```python
from build123d import *

# Parameters (mm, degrees)
EXTRUDE_1_DEPTH     = 2.5
CUT_EXTRUDE_1_DEPTH = 1
CUT_EXTRUDE_2_DEPTH = 3.8
CUT_EXTRUDE_3_DEPTH = 1


with BuildPart() as part:
    # Sketch 1 → Extrude 1 (new body)
    with BuildSketch(Plane(origin=(0, 0, 0), x_dir=(1, 0, 0), z_dir=(0, 1, 0))):
        Polygon((-33.25966317, -13.776603565), (-13.776603565, -33.25966317), (13.776603565, -33.25966317), (33.25966317, -13.776603565), (33.25966317, 13.776603565), (13.776603565, 33.25966317), (-13.776603565, 33.25966317), (-33.25966317, 13.776603565), align=None)
        Polygon((-13.27954729, -32.05966317), (13.27954729, -32.05966317), (32.05966317, -13.27954729), (32.05966317, 13.27954729), (13.27954729, 32.05966317), (-13.27954729, 32.05966317), (-32.05966317, 13.27954729), (-32.05966317, -13.27954729), align=None, mode=Mode.SUBTRACT)
        Polygon((-32.05966317, -13.27954729), (-13.27954729, -32.05966317), (13.27954729, -32.05966317), (32.05966317, -13.27954729), (32.05966317, 13.27954729), (13.27954729, 32.05966317), (-13.27954729, 32.05966317), (-32.05966317, 13.27954729), align=None)
        Polygon((-12.782491015, -30.85966317), (12.782491015, -30.85966317), (30.85966317, -12.782491015), (30.85966317, 12.782491015), (12.782491015, 30.85966317), (-12.782491015, 30.85966317), (-30.85966317, 12.782491015), (-30.85966317, -12.782491015), align=None, mode=Mode.SUBTRACT)
        Polygon((-30.85966317, -12.782491015), (-12.782491015, -30.85966317), (12.782491015, -30.85966317), (30.85966317, -12.782491015), (30.85966317, 12.782491015), (12.782491015, 30.85966317), (-12.782491015, 30.85966317), (-30.85966317, 12.782491015), align=None)
    extrude(amount=EXTRUDE_1_DEPTH)

    # Sketch 2 → Cut-Extrude 1 (cut)
    with BuildSketch(Plane(origin=(0, 2.5, 0), x_dir=(1, 0, 0), z_dir=(0, 1, 0))):
        Polygon((13.317383446, -32.151007731), (32.151007731, -13.317383446), (32.151007731, 13.317383446), (13.317383446, 32.151007731), (-13.317383446, 32.151007731), (-32.151007731, 13.317383446), (-32.151007731, -13.317383446), (-13.317383446, -32.151007731), align=None)
        Polygon((12.820327171, -30.951007731), (30.951007731, -12.820327171), (30.951007731, 12.820327171), (12.820327171, 30.951007731), (-12.820327171, 30.951007731), (-30.951007731, 12.820327171), (-30.951007731, -12.820327171), (-12.820327171, -30.951007731), align=None, mode=Mode.SUBTRACT)
    extrude(amount=-CUT_EXTRUDE_1_DEPTH, mode=Mode.SUBTRACT)

    # Sketch 4 → Cut-Extrude 2 (cut)
    with BuildSketch(Plane(origin=(0, 2.5, 0), x_dir=(1, 0, 0), z_dir=(0, 1, 0))):
        Polygon((-12.320132754, -5.103166077), (-5.103166077, -12.320132754), (5.103166077, -12.320132754), (12.320132754, -5.103166077), (12.320132754, 5.103166077), (5.103166077, 12.320132754), (-5.103166077, 12.320132754), (-12.320132754, 5.103166077), align=None)
    extrude(amount=-CUT_EXTRUDE_2_DEPTH, mode=Mode.SUBTRACT)

    # Sketch 4_3 → Cut-Extrude 3 (cut)
    with BuildSketch(Plane(origin=(0, 2.5, 0), x_dir=(1, 0, 0), z_dir=(0, 1, 0))):
        Polygon((-14.320132754, -5.931593202), (-5.931593202, -14.320132754), (5.931593202, -14.320132754), (14.320132754, -5.931593202), (14.320132754, 5.931593202), (5.931593202, 14.320132754), (-5.931593202, 14.320132754), (-14.320132754, 5.931593202), align=None)
        Polygon((-5.517379639, -13.320132754), (5.517379639, -13.320132754), (13.320132754, -5.517379639), (13.320132754, 5.517379639), (5.517379639, 13.320132754), (-5.517379639, 13.320132754), (-13.320132754, 5.517379639), (-13.320132754, -5.517379639), align=None, mode=Mode.SUBTRACT)
    extrude(amount=-CUT_EXTRUDE_3_DEPTH, mode=Mode.SUBTRACT)


solid = part.part
```
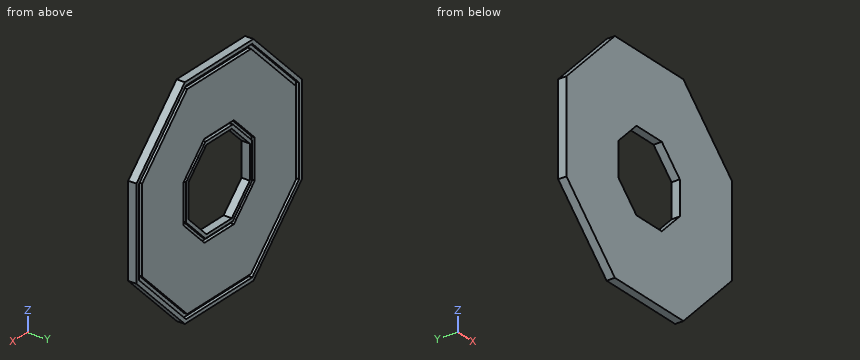
CAD build for the part. Positions are in the model's coordinates, mm. Give positions to 0.01 mm unless a question says otherwise; leave off trailing zeros. Order: outer loops, then holes, each group sorted by start corner. A loop starts at its lowest first (then second) coordinate and runs counter-clockwise, first axis right, second up.
(1) Flat gauge pin, fed straight in: pin 1 (2 mm diameter, centred on x = 24, z = -22, fed in from -Y). Where does the tip first touch, or does it go through?
(2) Saw through at B-B, the plane y = 2.1. State how many separate pieces and enclosed holes the cut face has, then the cut area to 3 significant figures.
(3) Saw through at C-C, the plane z = 7. Give the cut face in (x, y), then the cut area to 3 significant figures.
(4) Drill centre lines: L1, parallel to X at y = 1.45, z = 3; L2, parallel to Z at x = -17, y = 2.05; L3, parallel to X at y = 1.65, z = 24.5. Where is each one in solid material? Low to high.
(5) Saw through at A-A, the plane x = 7.5. Give the cut face in (y, z).
(6) Saw through at D-D, the plane x = 26. Give the cut face in (y, z).
Results found:
1. pin 1: stops at y = 0
2. separate pieces: 3
2. enclosed holes: 3
2. area: 2,820 mm2
3. outline: (-33.26, 0) - (-10.42, 0) - (-10.42, 2.5) - (-11.84, 2.5) - (-11.84, 1.5) - (-13.25, 1.5) - (-13.25, 2.5) - (-30.95, 2.5) - (-30.95, 1.5) - (-32.15, 1.5) - (-32.15, 2.5) - (-33.26, 2.5) - close; (10.42, 0) - (33.26, 0) - (33.26, 2.5) - (32.15, 2.5) - (32.15, 1.5) - (30.95, 1.5) - (30.95, 2.5) - (13.25, 2.5) - (13.25, 1.5) - (11.84, 1.5) - (11.84, 2.5) - (10.42, 2.5) - close
3. area: 109 mm2
4. L1: x = -33.26 to -12.32, 12.32 to 33.26
4. L2: z = -30.04 to -28.47, -26.77 to 26.77, 28.47 to 30.04
4. L3: x = -22.54 to -20.97, -19.27 to 19.27, 20.97 to 22.54
5. outline: (0, -33.26) - (2.5, -33.26) - (2.5, -32.15) - (1.5, -32.15) - (1.5, -30.95) - (2.5, -30.95) - (2.5, -12.75) - (1.5, -12.75) - (1.5, -11.34) - (2.5, -11.34) - (2.5, -9.92) - (0, -9.92) - close; (0, 9.92) - (2.5, 9.92) - (2.5, 11.34) - (1.5, 11.34) - (1.5, 12.75) - (2.5, 12.75) - (2.5, 30.95) - (1.5, 30.95) - (1.5, 32.15) - (2.5, 32.15) - (2.5, 33.26) - (0, 33.26) - close
6. outline: (0, -21.04) - (2.5, -21.04) - (2.5, -19.47) - (1.5, -19.47) - (1.5, -17.77) - (2.5, -17.77) - (2.5, 17.77) - (1.5, 17.77) - (1.5, 19.47) - (2.5, 19.47) - (2.5, 21.04) - (0, 21.04) - close
